Print and shaded views of the part. All mm, measured from the part's lowest x, y and z. A direction names the side the tool comes from. Coordinates: 2 decimals unless noted, no trailing zeros. Order: outer loops, then holes, each group sorted by start corner. A loop starts at its lowest first (then second) coordinate and runs counter-clockwise, first axis right, second up.
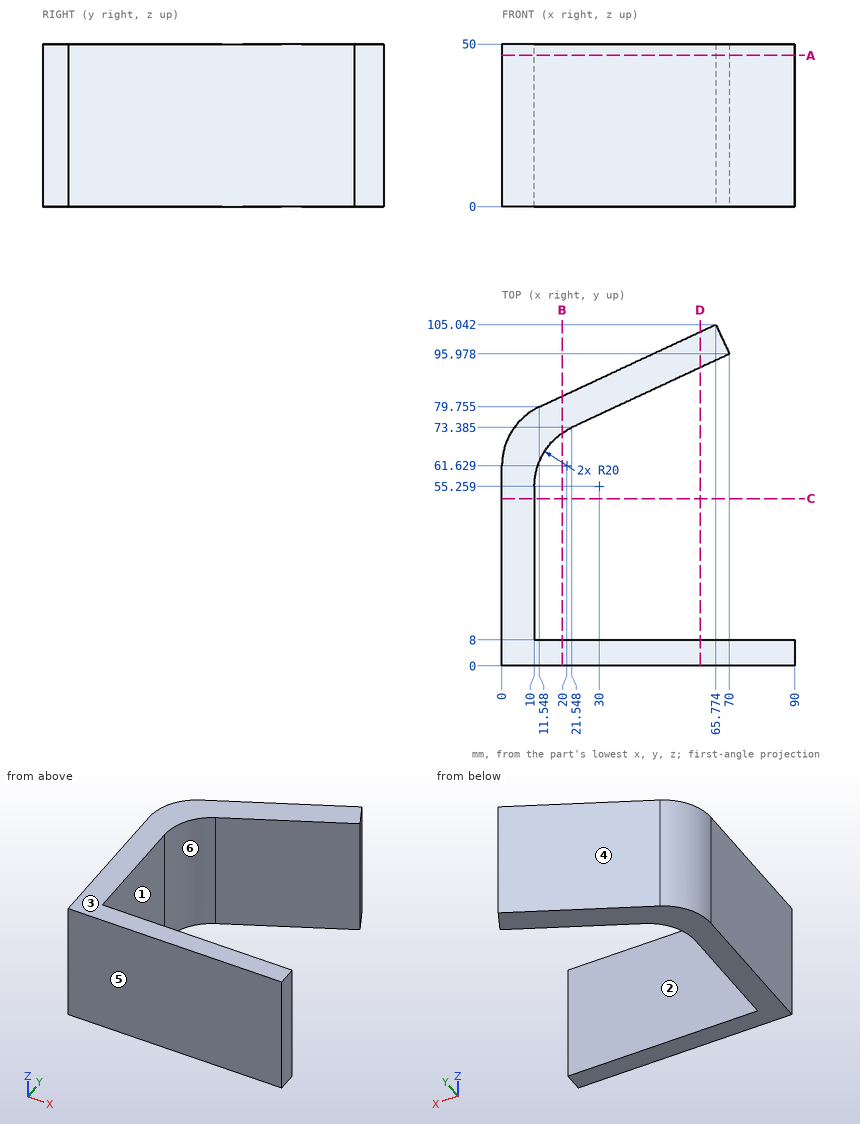
Q1. Cut at D-D, the plane x = 61. List the corners of the cut face in (y, z) (1 decimal).
Established:
outline: (0, 0) - (8, 0) - (8, 50) - (0, 50) - close; (91.8, 0) - (102.8, 0) - (102.8, 50) - (91.8, 50) - close
Q2. Cut at A-A, the plane z = 46.5. List the corners of the cut face in (x, y) (1 decimal).
Established:
outline: (0, 0) - (90, 0) - (90, 8) - (10, 8) - (10, 55.3) arc R20 cw to (21.5, 73.4) - (70, 96) - (65.8, 105) - (11.5, 79.8) arc R20 ccw to (0, 61.6) - close
Q3. Cut at B-B, the plane x = 18.5. List the corners of the cut face in (y, z).
Established:
outline: (0, 0) - (8, 0) - (8, 50) - (0, 50) - close; (71.62, 0) - (83, 0) - (83, 50) - (71.62, 50) - close
Q4. Drop flat-ended pins along their axis: P1, Ø1.5, axis at x = 29, z = 41, coming from the +Y side; P2, Ø1, axis at y = 90, z = 17, coming from the -X side (1 decimal); P3, Ø1.5, axis at y = 18.5, z = 43, coming from the +X side; P4, Ø10, axis at y = 53, z = 6, coming from the -X side. Give the stop position or say it passes through.
Established:
P1: stops at y = 88.24
P2: stops at x = 32.4
P3: stops at x = 10
P4: stops at x = 0
Q5. Cut at C-C, the plane y = 51.5. List the corners of the cut face in (x, z).
Established:
outline: (0, 0) - (10, 0) - (10, 50) - (0, 50) - close
Q6. Probe line 1 (X direction, y = 24.5, z = 31); line 2 (Y direction, x = 78, z = 44); line 3 (Y direction, x = 46, z = 35). List the from-to ranges inside material, lowest first.
Established:
line 1: x = 0 to 10
line 2: y = 0 to 8
line 3: y = 0 to 8, 84.79 to 95.82
Q7. Which spindle directions (+Z, -Z, +X, -X, +Y, -Y) get a long thin tool onto all of the face, cutting with end or side? Do the marked faces 5 and 6. Say none if no direction does.
Established:
face 5: +Z, -Z, +X, -X, -Y
face 6: +Z, -Z, +X
Q8. Mould opens along Y. For the marked faces 1, 2, 3 and 4 say: pulls with the +Y half, pulls with the -Y half, needs draft (parallel to the pull), parting line crosses it, or undercut.
Established:
face 1: undercut
face 2: undercut
face 3: needs draft
face 4: pulls with the +Y half
